Build history of the part. All positions in model axes, mm. A direction names the side the tool comes from. Give positions to 0.01 mm unless a question says otherwise; leave off trailing zeros. Write each loop counter-clockwise with the first axis right and the second up, starting at its lowest first coordinate (ties: lowest second). Pieces come first, ordered by that corner, then holes. Notation, with made-up numbers: (-16, -34.75) -> (1, -34.75) arc R22 ccw to (1, -26.75) -> close; hole circle Ø7 at (-21.5, 11.25). An arc over 180 degrees is marked (long way). Write item = value, one per line. Start each with the question number.
Q1. Wall check: line 1 (Y direction, x = 0.6, z = -12.7); line 2 (X direction, y = 18.5, z = -9.75); line 3 (Z direction, x = 15, y = 34). Give the ranges that are in metal, low to high.
Q2. Drop flat-ended pins along their axis: P1, Ø3, axis at y = 7, z = -20, coming from the +X side; P2, Ø12, axis at x = 38, y = 32.5, coming from the -Z side. Give the stop position or say it passes through.
Q3. Saw through at D-D, the plane z = -17.25. List the corners of the cut face in (x, y), then the cut area to 3 significant figures.
Q4. Mould opens along Z. For faces 1 (the face through (38, 31, -1.214)), 2 (the face through (0.6, 49.33, -13.31)), 3 (the face through (38, 63.5, -1)) say: pulls with the +Z half, pulls with the -Z half, needs draft (parallel to the pull), parting line crosses it, or undercut.
Q5. Tool access for faces 4 (the face through (39, 31, 0)), 5 (the face through (1.214, 31, -13)): list every direction of +Z, -Z, +X, -X, +Y, -Y with a clear straight run to the whole face (end or side of a thin tool).
Q6. Saw through at C-C, the plane x = 22.5. List the corners of the cut face in (y, z).
Q7. Saw through at A-A, the plane z = -12.7. List the corners of the cut face in (x, y).
Q8. Saw through at B-B, the plane y = 11.43. List the corners of the cut face in (x, z).
from build123d import *

# Parameters (mm, degrees)
BOSS_EXTRUDE1_DEPTH = 63.5
SKETCH3_R           = 2.8067
CUT_EXTRUDE1_DEPTH  = 2.54


with BuildPart() as part:
    # Sketch2 → Boss-Extrude1 (new body)
    with BuildSketch(Plane(origin=(0, 0, 0), x_dir=(1, 0, 0), z_dir=(0, 1, 0))):
        Polygon((0, 0), (0, 25.4), (1.21412, 25.4), (1.21412, 1.21412), (76.2, 1.21412), (76.2, 0), align=None)
    extrude(amount=BOSS_EXTRUDE1_DEPTH)

    # Sketch3 → Cut-Extrude1 (cut)
    with BuildSketch(Plane.ZY):
        with Locations((-12.7, 52.07)):
            Circle(SKETCH3_R)
        with Locations((-12.7, 11.43)):
            Circle(SKETCH3_R)
    extrude(amount=-CUT_EXTRUDE1_DEPTH, mode=Mode.SUBTRACT)


solid = part.part
Report:
q1.line_1 = 0 to 8.62, 14.24 to 49.26, 54.88 to 63.5
q1.line_2 = 0 to 1.21
q1.line_3 = -1.21 to 0
q2.P1 = 1.21
q2.P2 = -1.21
q3.outline = (0, 0) -> (1.21, 0) -> (1.21, 63.5) -> (0, 63.5) -> close
q3.area = 77.1 mm2
q4.face_1 = pulls with the -Z half
q4.face_2 = undercut
q4.face_3 = needs draft
q5.face_4 = +Z, +X, -X, +Y, -Y
q5.face_5 = -Z, +X, +Y, -Y
q6.outline = (0, -1.21) -> (63.5, -1.21) -> (63.5, 0) -> (0, 0) -> close
q7.outline = (0, 0) -> (1.21, 0) -> (1.21, 8.62) -> (0, 8.62) -> close; (0, 14.24) -> (1.21, 14.24) -> (1.21, 49.26) -> (0, 49.26) -> close; (0, 54.88) -> (1.21, 54.88) -> (1.21, 63.5) -> (0, 63.5) -> close
q8.outline = (0, -25.4) -> (1.21, -25.4) -> (1.21, -15.51) -> (0, -15.51) -> close; (0, -9.89) -> (1.21, -9.89) -> (1.21, -1.21) -> (76.2, -1.21) -> (76.2, 0) -> (0, 0) -> close
